Part model, mm, in its own coordinate system. A direction names the side the tool comes from. Round coordinates to 2 decimals unless told otherwise and drop trailing zeros. Order: outer loops, then holes, each group sorted by start corner. A loop starts at its lowest first (then second) coordinate and runs counter-clockwise, first axis right, second up. Notation, with made-up numbers: (-8.5, 32.25) - (12.5, 32.25) arc R17 ccw to (12.5, 52.25) - close; hole circle Ø11 at (-38, 9). An arc over 180 degrees is marked (long way). Return JSON: item names as keys, results as strings. Group by question number.
Item 1: Saw through at C-C on y = -31. List the corners of the cut face in (x, z).
Item 2: Probe probe 1 along Z at (x, y) = (21, -20); probe 2 along Y at (x, z) = (20, -4). List the from-to ranges inside material, lowest first.
Item 3: Tool access for faces 1 (the face through (0, 11, -17)), 2 (the face through (18.796, 11, -17)), 3 (the face through (10, -27, -6.35)): list every direction of +Z, -Z, +X, -X, +Y, -Y with a clear straight run to the whole face (end or side of a thin tool).
Item 4: Drop flat-ended pins along their axis: pin 1 (5 mm diameter, centred on x = -7, y = -5.5, fed in from -Z); pin 2 (10 mm diameter, centred on x = 4, z = -14, fed in from +Y); pin 3 (12 mm diameter, centred on x = 12.5, z = -22.5, fed in from -Y); pin 4 (12 mm diameter, centred on x = 13, y = 3, fed in from +Z). Give the stop position or say it passes through.
Item 5: Saw through at B-B on x = 15.5. List the corners of the cut face in (y, z).
Item 6: Saw through at A-A on z = -3. List the corners of the cut face in (x, y).
Item 7: Saw through at D-D on x = 27. List the corners of the cut face in (y, z).
```python
from build123d import *

# Parameters (mm, degrees)
BOSS_EXTRUDE1_DEPTH = 18.796
SKETCH2_W           = 6.35
SKETCH2_H           = 47.838946371
BOSS_EXTRUDE2_DEPTH = 25.4
SKETCH3_W           = 6.35
SKETCH3_H           = 47.838946371
BOSS_EXTRUDE3_DEPTH = 25.4


with BuildPart() as part:
    # Sketch1 → Boss-Extrude1 (new body)
    with BuildSketch(Plane(origin=(0, 0, 0), x_dir=(0, 0, -1), z_dir=(1, 0, 0))):
        Polygon((0, 0), (0, -50.8), (6.35, -50.8), (6.35, -2.961053629), (33.267994604, 19.625825715), (29.186293283, 24.490207929), align=None)
    extrude(amount=BOSS_EXTRUDE1_DEPTH)

    # Sketch2 → Boss-Extrude2 (add)
    with BuildSketch(Plane(origin=(18.796, 0, 0), x_dir=(0, 0, -1), z_dir=(1, 0, 0))):
        with Locations((3.175, -26.880526815)):
            Rectangle(SKETCH2_W, SKETCH2_H)
    extrude(amount=BOSS_EXTRUDE2_DEPTH)

    # Sketch3 → Boss-Extrude3 (add)
    with BuildSketch(Plane.ZY):
        with Locations((-3.175, -26.880526815)):
            Rectangle(SKETCH3_W, SKETCH3_H)
    extrude(amount=BOSS_EXTRUDE3_DEPTH)


solid = part.part
```
Filled in:
{
 "1": {"outline": "(-25.4, -6.35) - (44.2, -6.35) - (44.2, 0) - (-25.4, 0) - close"},
 "2": {"probe 1": "z = -6.35 to 0", "probe 2": "y = -50.8 to -2.96"},
 "3": {"face 1": "+Z, -Z, -X, +Y", "face 2": "+Z, -Z, +X, +Y", "face 3": "-Z, +X, -X, -Y"},
 "4": {"pin 1": "stops at z = -6.35", "pin 2": "stops at y = 15.94", "pin 3": "stops at y = 5.56", "pin 4": "stops at z = 0"},
 "5": {"outline": "(-50.8, -6.35) - (-2.96, -6.35) - (19.63, -33.27) - (24.49, -29.19) - (0, 0) - (-50.8, 0) - close"},
 "6": {"outline": "(-25.4, -50.8) - (44.2, -50.8) - (44.2, -2.96) - (18.8, -2.96) - (18.8, 2.52) - (0, 2.52) - (0, -2.96) - (-25.4, -2.96) - close"},
 "7": {"outline": "(-50.8, -6.35) - (-2.96, -6.35) - (-2.96, 0) - (-50.8, 0) - close"}
}
